Can you work these out from the model? Positions are in its coordinate system, mm. A direction names the side the tool comes from. Round coordinates to 2 decimals unless told otherwise and drop trailing zeros. Order: outer loops, then holes, each group sorted by start corner. A loop starts at its lowest first (then second) coordinate and runs counter-clockwise, first axis right, second up. Notation, with made-up numbers: (64.5, 68.5) -> (81.5, 68.5) arc R15 cw to (81.5, 74.5) -> close; hole circle Ø5 at (13.5, 67.5). An arc over 180 degrees is marked (long way). Use a Markdown table: item, result. Add a question column.
Q1. If we section it at B-B on x = -34.5: List the corners of the cut face in (y, z) for me, plus the area to 3 significant figures.
Q2. If we section it at C-C on y = -13: List the corners of the cut face in (x, z) for me.
Q3. For faces 4 (the face through (-1, 0, 24)), 5 (the face through (25.672, -9.528, 13.054)), 6 (the face through (-40.528, 2.391, 2.423)), 7 (the face through (38.5, 4, 3)), which set-ups out of +Z, -Z, +X, -X, +Y, -Y let a thin tool reach every point of the face, with its end or its side?
Q4. If we section it at D-D on x = 17: List the corners of the cut face in (y, z) for me, plus the area to 3 significant figures.
Q5. I'm going to push flat-ended pins straight in: pin 1 Ø2 at (x, z) = (25.5, 20) entering from -Y; pin 2 Ø2 at (x, z) = (25, 12) entering from -Y; pin 3 Ø2 at (y, z) = (3.5, 21) entering from +X. Where does each tip first touch, or does it pass through?
Q6. If we section it at A-A on z = 21: List the corners of the cut face in (x, y) for me.
Q7. I need wall thicknesses on line 1 along Y through (x, z) = (-40.7, 21); line 2 along Z through (x, y) = (25, -8); line 3 along Y through (x, z) = (-18, 10.75). Which ranges of each line are inside material? Lowest first, please. Write a range as [from, to].
Q8. We'd pull the mould along X, two halves only. Please class faces 1 (the face through (-38.5, 3, 21)), 2 (the face through (-25, -7.5, 12)), 3 (the face through (40.528, 2.391, 2.423)): +X half, -X half, draft (parallel to the pull), parting line (faces both ways), or undercut.
```python
from build123d import *

# Parameters (mm, degrees)
SKETCH1_W           = 85
SKETCH1_H           = 23
BOSS_EXTRUDE1_DEPTH = 24
SKETCH3_R           = 1.25
CUT_EXTRUDE1_DEPTH  = 4
SKETCH4_R           = 1.25
CUT_EXTRUDE2_DEPTH  = 4
SKETCH5_R           = 2
BOSS_EXTRUDE3_DEPTH = 10


with BuildPart() as part:
    # Sketch1 → Boss-Extrude1 (new body)
    with BuildSketch(Plane.XY):
        Rectangle(SKETCH1_W, SKETCH1_H)
    extrude(amount=BOSS_EXTRUDE1_DEPTH)

    # Sketch3 → Cut-Extrude1 (cut)
    with BuildSketch(Plane.XZ.offset(11.5)):
        with Locations((-25, 12)):
            Circle(SKETCH3_R)
        with Locations((25, 12)):
            Circle(SKETCH3_R)
    extrude(amount=-CUT_EXTRUDE1_DEPTH, mode=Mode.SUBTRACT)

    # Sketch4 → Cut-Extrude2 (cut)
    with BuildSketch(Plane(origin=(42.5, 0, 0), x_dir=(0, 0, -1), z_dir=(1, 0, 0))):
        with Locations((-3, 3.5)):
            Circle(SKETCH4_R)
        with Locations(Location((-21, 3.5, 0), (0, 0, 180))):
            Circle(SKETCH4_R)
    cut_extrude2 = extrude(amount=-CUT_EXTRUDE2_DEPTH, mode=Mode.SUBTRACT)

    # Mirror1: Cut-Extrude2 across plane
    add(cut_extrude2.mirror(Plane(origin=(0, 0, 0), x_dir=(0, 0, 1), z_dir=(1, 0, 0))), mode=Mode.SUBTRACT)

    # Sketch5 → Boss-Extrude3 (add)
    with BuildSketch(Plane.XZ.offset(11.5)):
        with Locations(Location((-34.5, 12, 0), (0, 0, 180))):
            Circle(SKETCH5_R)
    extrude(amount=BOSS_EXTRUDE3_DEPTH)


solid = part.part
```
Answer below:
| question | item | result |
|---|---|---|
| 1 | outline | (-21.5, 10) -> (-11.5, 10) -> (-11.5, 0) -> (11.5, 0) -> (11.5, 24) -> (-11.5, 24) -> (-11.5, 14) -> (-21.5, 14) -> close |
| 1 | area | 592 mm² |
| 2 | outline | circle Ø4 at (-34.5, 12) |
| 3 | face 4 | +Z, +X, -X, +Y, -Y |
| 3 | face 5 | -Y |
| 3 | face 6 | -X |
| 3 | face 7 | +X |
| 4 | outline | (-11.5, 0) -> (11.5, 0) -> (11.5, 24) -> (-11.5, 24) -> close |
| 4 | area | 552 mm² |
| 5 | pin 1 | y = -11.5 |
| 5 | pin 2 | y = -7.5 |
| 5 | pin 3 | x = 38.5 |
| 6 | outline | (-42.5, -11.5) -> (42.5, -11.5) -> (42.5, 2.25) -> (38.5, 2.25) -> (38.5, 4.75) -> (42.5, 4.75) -> (42.5, 11.5) -> (-42.5, 11.5) -> (-42.5, 4.75) -> (-38.5, 4.75) -> (-38.5, 2.25) -> (-42.5, 2.25) -> close |
| 7 | line 1 | [-11.5, 2.25], [4.75, 11.5] |
| 7 | line 2 | [0, 10.75], [13.25, 24] |
| 7 | line 3 | [-11.5, 11.5] |
| 8 | face 1 | -X half |
| 8 | face 2 | undercut |
| 8 | face 3 | draft |
